Check sheet for the modelled part. Datum: model origin and axes. Units: mm. A direction names the side the tool comes from. Round coordinates to 2 decimals unless told otherwise and drop trailing zeros. Order: outer loops, then holes, each group sorted by start corner. A loop starts at its lowest first (then second) coordinate and runs counter-clockwise, first axis right, second up. Notation, with made-up numbers: (-9.75, 37) -> (11.25, 37) arc R22 cw to (11.25, 61) -> close; hole circle Ø10 at (3.25, 51). An arc over 180 degrees is marked (long way). Answer in a Markdown table with one row per item.
```python
from build123d import *

# Parameters (mm, degrees)
SKETCH_1_R          = 52
SKETCH_1_R_2        = 1.55
SKETCH_1_R_3        = 2.05
SKETCH_1_R_4        = 13
EXTRUDE_1_DEPTH     = 3
FILLET_1_R          = 3
SKETCH_2_R          = 4.6
CUT_EXTRUDE_1_DEPTH = 1.3
SKETCH_3_R          = 68.655116319
SKETCH_3_R_2        = 50
CUT_EXTRUDE_2_DEPTH = 10


with BuildPart() as part:
    # 草图1 → 凸台-拉伸1 (new body)
    with BuildSketch(Plane.XY):
        Circle(SKETCH_1_R)
        with Locations((46, 0)):
            Circle(SKETCH_1_R_2, mode=Mode.SUBTRACT)
        with Locations((23, -39.837168574)):
            Circle(SKETCH_1_R_2, mode=Mode.SUBTRACT)
        with Locations((-23, -39.837168574)):
            Circle(SKETCH_1_R_2, mode=Mode.SUBTRACT)
        with Locations((-46, 0)):
            Circle(SKETCH_1_R_2, mode=Mode.SUBTRACT)
        with Locations((-23, 39.837168574)):
            Circle(SKETCH_1_R_2, mode=Mode.SUBTRACT)
        with Locations((23, 39.837168574)):
            Circle(SKETCH_1_R_2, mode=Mode.SUBTRACT)
        with Locations((0, 22.5)):
            Circle(SKETCH_1_R_3, mode=Mode.SUBTRACT)
        with Locations((19.485571585, 11.25)):
            Circle(SKETCH_1_R_3, mode=Mode.SUBTRACT)
        with Locations((19.485571585, -11.25)):
            Circle(SKETCH_1_R_3, mode=Mode.SUBTRACT)
        with Locations((0, -22.5)):
            Circle(SKETCH_1_R_3, mode=Mode.SUBTRACT)
        with Locations((-19.485571585, -11.25)):
            Circle(SKETCH_1_R_3, mode=Mode.SUBTRACT)
        with Locations((-19.485571585, 11.25)):
            Circle(SKETCH_1_R_3, mode=Mode.SUBTRACT)
        Circle(SKETCH_1_R_4, mode=Mode.SUBTRACT)
        with BuildLine():
            Line((14, 0), (37.606451003, 13.629190841))
            ThreePointArc((37.606451003, 13.629190841), (40, 0), (37.606451003, -13.629190841))
            Line((37.606451003, -13.629190841), (14, 0))
        make_face(mode=Mode.SUBTRACT)
        with BuildLine():
            Line((7, -12.124355653), (7, -39.382737335))
            ThreePointArc((7, -39.382737335), (20, -34.641016151), (30.606451003, -25.753546494))
            Line((30.606451003, -25.753546494), (7, -12.124355653))
        make_face(mode=Mode.SUBTRACT)
        with BuildLine():
            Line((-7, -12.124355653), (-30.606451003, -25.753546494))
            ThreePointArc((-30.606451003, -25.753546494), (-20, -34.641016151), (-7, -39.382737335))
            Line((-7, -39.382737335), (-7, -12.124355653))
        make_face(mode=Mode.SUBTRACT)
        with BuildLine():
            Line((-14, 0), (-37.606451003, 13.629190841))
            ThreePointArc((-37.606451003, 13.629190841), (-40, 0), (-37.606451003, -13.629190841))
            Line((-37.606451003, -13.629190841), (-14, 0))
        make_face(mode=Mode.SUBTRACT)
        with BuildLine():
            Line((-7, 12.124355653), (-7, 39.382737335))
            ThreePointArc((-7, 39.382737335), (-20, 34.641016151), (-30.606451003, 25.753546494))
            Line((-30.606451003, 25.753546494), (-7, 12.124355653))
        make_face(mode=Mode.SUBTRACT)
        with BuildLine():
            Line((7, 12.124355653), (30.606451003, 25.753546494))
            ThreePointArc((30.606451003, 25.753546494), (20, 34.641016151), (7, 39.382737335))
            Line((7, 39.382737335), (7, 12.124355653))
        make_face(mode=Mode.SUBTRACT)
    extrude(amount=EXTRUDE_1_DEPTH)

    # 圆角1
    fillet_1_edges = [part.edges().sort_by_distance(p)[0] for p in [
        (7, 39.382737335, 1.5),
        (7, 12.124355653, 1.5),
        (30.606451003, 25.753546494, 1.5),
        (14, 0, 1.5),
        (37.606451003, -13.629190841, 1.5),
        (37.606451003, 13.629190841, 1.5),
        (30.606451003, -25.753546494, 1.5),
        (7, -12.124355653, 1.5),
        (7, -39.382737335, 1.5),
        (-7, -39.382737335, 1.5),
        (-7, -12.124355653, 1.5),
        (-30.606451003, -25.753546494, 1.5),
        (-37.606451003, -13.629190841, 1.5),
        (-14, 0, 1.5),
        (-37.606451003, 13.629190841, 1.5),
        (-30.606451003, 25.753546494, 1.5),
        (-7, 12.124355653, 1.5),
        (-7, 39.382737335, 1.5),
    ]]
    fillet(fillet_1_edges, radius=FILLET_1_R)

    # 草图2 → 切除-拉伸1 (cut)
    with BuildSketch(Plane.XY.offset(3)):
        with Locations((-19.485571585, 11.25)):
            Circle(SKETCH_2_R)
        with Locations((0, 22.5)):
            Circle(SKETCH_2_R)
        with Locations((19.485571585, 11.25)):
            Circle(SKETCH_2_R)
        with Locations((19.485571585, -11.25)):
            Circle(SKETCH_2_R)
        with Locations((0, -22.5)):
            Circle(SKETCH_2_R)
        with Locations((-19.485571585, -11.25)):
            Circle(SKETCH_2_R)
    extrude(amount=-CUT_EXTRUDE_1_DEPTH, mode=Mode.SUBTRACT)

    # 草图3 → 切除-拉伸2 (cut)
    with BuildSketch(Plane.XY.offset(3)):
        Circle(SKETCH_3_R)
        Circle(SKETCH_3_R_2, mode=Mode.SUBTRACT)
    extrude(amount=-CUT_EXTRUDE_2_DEPTH, mode=Mode.SUBTRACT)


solid = part.part
```
(1) Section check B-B on x = -46. Record the boundary of the cut face in (y, z), plus the area to 3 significant figures.
Solutions:
| item | result |
|---|---|
| outline | (-19.6, 0) -> (-1.55, 0) -> (-1.55, 3) -> (-19.6, 3) -> close; (1.55, 0) -> (19.6, 0) -> (19.6, 3) -> (1.55, 3) -> close |
| area | 108 mm^2 |
(2) Draft check along X on faces 1 (the cylindrical face through (23.735, 9.488, 2.359)), 2 (the cylindrical face through (-20.12, -34.57, 1.48)), 3 (the cylindrical face through (47.69, 15.02, 1.52)). Enter one of: pulls with the +X half, pulls with the -X half, needs draft (parallel to the pull), parting line crosses it, or undercut.
Solutions:
| item | result |
|---|---|
| face 1 | undercut |
| face 2 | undercut |
| face 3 | parting line crosses it |
(3) Section check A-A on y = 0. Record the boundary of the cut face in (x, z).
Solutions:
| item | result |
|---|---|
| outline | (-50, 0) -> (-47.55, 0) -> (-47.55, 3) -> (-50, 3) -> close; (-44.45, 0) -> (-40, 0) -> (-40, 3) -> (-44.45, 3) -> close; (-17, 0) -> (-13, 0) -> (-13, 3) -> (-17, 3) -> close; (13, 0) -> (17, 0) -> (17, 3) -> (13, 3) -> close; (40, 0) -> (44.45, 0) -> (44.45, 3) -> (40, 3) -> close; (47.55, 0) -> (50, 0) -> (50, 3) -> (47.55, 3) -> close |
(4) Section check D-D on z = 1.2. Give the number of separate pieces and of enclosed holes in the cut face, plus the area to 3 significant figures.
Solutions:
| item | result |
|---|---|
| separate pieces | 1 |
| enclosed holes | 19 |
| area | 5,080 mm^2 |
(5) Section check C-C on y = 32. Record the boundary of the cut face in (x, z), plus the area to 3 significant figures.
Solutions:
| item | result |
|---|---|
| outline | (-38.42, 0) -> (-24, 0) -> (-24, 3) -> (-38.42, 3) -> close; (-7, 0) -> (7, 0) -> (7, 3) -> (-7, 3) -> close; (24, 0) -> (38.42, 0) -> (38.42, 3) -> (24, 3) -> close |
| area | 129 mm^2 |
(6) Tool access check on faces 4 (the cylindrical face through (-36.98, 11.93, 1.52)), 5 (the flat face through (21.5, -12.2, 1.7)). Record the directions out of +Z, -Z, +X, -X, +Y, -Y that give a thin tool (end or side, any length) a straight path to the whole face; none if there is none.
Solutions:
| item | result |
|---|---|
| face 4 | +Z, -Z |
| face 5 | +Z |
(7) Scan lines: probe 1 along Y at (x, z) = (0, 0.8); probe 2 along Y at (x, z) = (-26.5, 0.55); probe 3 along X at (y, z) = (25.5, 1). Record each from-to range of solid material in increasing order. Write a range as from..to.
Solutions:
| item | result |
|---|---|
| probe 1 | -50..-24.55, -20.45..-13, 13..20.45, 24.55..50 |
| probe 2 | -42.4..-29.96, -23.38..-7.22, 7.22..23.38, 29.96..42.4 |
| probe 3 | -43.01..-28.69, -7..7, 28.69..43.01 |
(8) Depth check by flat-ended pin: pin 1 Ø4.5 at (x, y) = (-19.49, -11.25) entering from +Z; pin 2 Ø1.5 at (y, z) = (38.5, 1.5) entering from +X. Enter the tip coordinate at first touch or a pass-through.
Solutions:
| item | result |
|---|---|
| pin 1 | z = 1.7 |
| pin 2 | x = 32.79 |
